Design review of the part built by this model. Coordinates are the model's own, in mm. Face numbers are marked on the shaded views. Give positions to 0.01 mm unless a question says otherwise; leave off trailing zeros. Loops run counter-clockwise (first coordinate to the right, second up) from the corner with the lowest first, then second, coordinate; pieces in that order, holes last. Notation, with made-up numbers: M 53,32 L 106,32 A18 cw 106,43 Z; hole C 0,16.5 d11. An arc over 180 degrees is marked long. Use a Markdown table: item, result. Add a question column.
(1) For probe 1 along X at (y, z) = (4.75, -106.5); probe 2 along Z at (x, y) = (23, 7); probe 3 along Y at (x, z) = (12, -13.5), list the stretches that pass through material, from the lowest coordinate up.
(2) Add section B-B, the plane x = 12.5. Give the boundary of the cut face in (y, z), then the cut area to 3 significant figures.
(3) Add section A-A, the plane z = -117.5. Give the boundary of the cut face in (x, y), then the cut area to 3 significant figures.
(4) Insertion check: pin 1 Ø2 at (x, z) = (16.5, -15.5) entering from +Y; pin 2 Ø1.5 at (x, y) = (-3, 3) entering from +Z; pin 3 Ø1.5 at (y, z) = (7, -68) entering from -X. Each pin has a flat end and moves straight along its axis. Give the tip position at first contact, or say it passes through.
(5) Draft analysis for pull direction X (two halves, no side actions). For the marked faces 1 and 2, state which applies: pulls with the +X half, pulls with the -X half, needs draft (parallel to the pull), parting line crosses it, or undercut.
(6) Add section C-C, the plane y = 7.5. Give the boundary of the cut face in (x, z), then the cut area to 3 significant figures.
(7) Add section D-D, the plane z = 37.5. Give the boundary of the cut face in (x, y), then the cut area to 3 significant figures.
Autodesk Inventor part; units mm, degrees
ref_plane "YZ Plane" through (0, 0, 0) normal (1, 0, 0) x (0, 1, 0)
ref_plane "XZ Plane" through (0, 0, 0) normal (0, 1, 0) x (-1, 0, 0)
ref_plane "XY Plane" through (0, 0, 0) normal (0, 0, 1) x (1, 0, 0)
sketch "Sketch1" plane through (0, 0, 0) normal (0, 0, 1) x (1, 0, 0)
  line L0 (0, 0) -> (30, 0)
  line L1 (30, 0) -> (30, 10)
  line L2 (30, 10) -> (0, 10)
  line L3 (0, 10) -> (0, 0)
  dimension "d0" = 30
  dimension "d1" = 10
extrude "Extrusion1" add sketch "Sketch1" along normal blind 100
sketch "Sketch2" plane through (0, 0, 0) normal (0, 0, -1) x (-1, 0, 0)
  line L0 (0, 10) -> (0, 0)
  line L1 (-30, 10) -> (0, 10)
  arc A0 (0, 0) -> (-5, 5) centre (0, 5) ccw
  line L2 (-30, 0) -> (-30, 10)
  line L3 (-30, 5) -> (-5, 5)
  line L4 (0, 0) -> (-30, 0)
  line L5 (-30, 0) -> (-30, 5)
extrude "Extrusion2" add sketch "Sketch2" along normal blind 100 contours A0 L0 | L0 L4 L2 L3 A0
sketch "Sketch3" plane through (0, 0, -100) normal (0, 0, -1) x (-1, 0, 0)
  line L0 (-30, 10) -> (0, 10)
  line L1 (0, 10) -> (-5, 5)
  arc A0 (0, 0) -> (-5, 5) centre (0, 5) ccw
  line L2 (0, 10) -> (5, 5)
  line L3 (-30, 0) -> (-30, 10)
  line L4 (-30, 5) -> (-5, 5)
  line L5 (5, 5) -> (5, 0)
  line L6 (5, 0) -> (-30, 0)
  line L7 (-30, 0) -> (-30, 5)
extrude "Extrusion3" add sketch "Sketch3" along normal blind 100 contours L2 A0 L6 L3 L4 L1
sketch "Sketch4" plane through (0, 0, 100) normal (0, 0, 1) x (1, 0, 0)
  line L0 (30, 5) -> (5, 5)
  line L1 (30, 0) -> (30, 10)
  arc A0 (30, 0) -> (30, 10) centre (30, 5) ccw
  line L2 (30, 10) -> (30, 0)
  point P0 (0, 0)
extrude "Extrusion4" add sketch "Sketch4" against normal up to surface (100 mm away)
sketch "Sketch5" plane through (0, 0, 0) normal (0, 0, -1) x (-1, 0, 0)
  line L0 (-30, 10) -> (0, 10)
  line L1 (-32.5, 0) -> (-27.5, 0)
  line L2 (-27.5, 0) -> (-27.5, 10)
  line L3 (-27.5, 10) -> (-32.5, 10)
  line L4 (-32.5, 10) -> (-32.5, 0)
  line L5 (-30, 5) -> (-5, 5)
  line L6 (-32.5, 0) -> (-27.5, 10) construction
  line L7 (-27.5, 0) -> (-32.5, 10) construction
  point P0 (0, 0)
  dimension "d10" = 5
extrude "Extrusion5" add sketch "Sketch5" along normal blind 100
sketch "Sketch6" plane through (0, 0, -200) normal (0, 0, -1) x (-1, 0, 0)
  line L0 (-5, 5) -> (-30, 5)
  arc A0 (-30, 10) -> (-30, 0) centre (-30, 5) ccw
  line L1 (-30, 10) -> (0, 10)
  line L2 (-30, 5) -> (-30, 0)
  line L3 (-30, 10) -> (-30, 0)
  point P0 (0, 0)
extrude "Extrusion6" add sketch "Sketch6" against normal up to surface (100 mm away)
properties part number "edges_3DPrint"
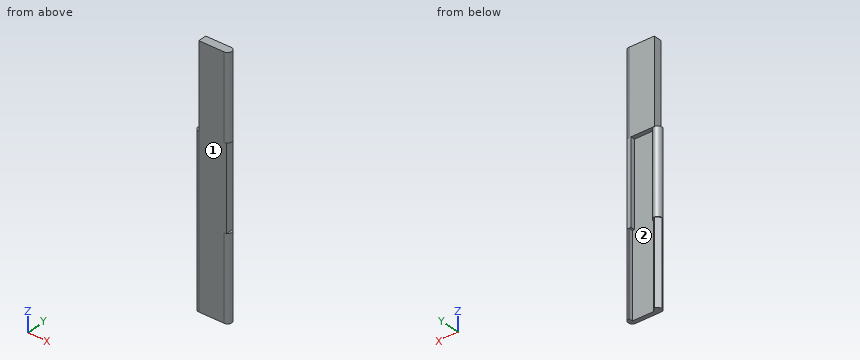
Established:
| question | item | result |
|---|---|---|
| 1 | probe 1 | -4.99 to 34.99 |
| 1 | probe 2 | 0 to 100 |
| 1 | probe 3 | 0 to 5 |
| 2 | outline | M 0,-200 L 5,-200 L 5,0 L 10,0 L 10,100 L 0,100 Z |
| 2 | area | 2,000 mm^2 |
| 3 | outline | M -5,5 A5 ccw 0,0 L 30,0 A5 ccw 30,10 L 30,5 L 5,5 L 0,10 Z |
| 3 | area | 234 mm^2 |
| 4 | pin 1 | y = 5 |
| 4 | pin 2 | z = 0 |
| 4 | pin 3 | x = -4.84 |
| 5 | face 1 | needs draft |
| 5 | face 2 | undercut |
| 6 | outline | M -4.33,-100 L -2.5,-100 L -2.5,-200 L 2.5,-200 L 2.5,-100 L 4.33,-100 L 4.33,0 L 27.5,0 L 27.5,-100 L 30,-100 L 30,-200 L 34.33,-200 L 34.33,-100 L 32.5,-100 L 32.5,0 L 34.33,0 L 34.33,100 L 0,100 L 0,0 L -4.33,0 Z |
| 6 | area | 5,730 mm^2 |
| 7 | outline | M 0,0 L 30,0 A5 ccw 30,10 L 0,10 Z |
| 7 | area | 339 mm^2 |
